from build123d import *

# Parameters (mm, degrees)
SKETCH1_W               = 100
SKETCH1_H               = 55
BOSS_EXTRUDE1_DEPTH     = 4
F_6_CLEARANCE_HOLE1_D   = 4.3053
SKETCH4_R               = 26
CUT_EXTRUDE1_DEPTH      = 1.5
BOSS_EXTRUDE2_DEPTH     = 2
CUT_EXTRUDE2_REACH      = 59.204
SKETCH7_W               = 22.5
SKETCH7_H               = 7
MIRROR2_COPY_1_DEPTH    = 2
MIRROR2_COPY_2_REACH    = 59.204
MIRROR2_COPY_2_SKETCH_W = 22.5
MIRROR2_COPY_2_SKETCH_H = 7
FILLET1_R               = 5


with BuildPart() as part:
    # Sketch1 → Boss-Extrude1 (new body)
    with BuildSketch(Plane(origin=(0, 0, 0), x_dir=(1, 0, 0), z_dir=(0, 1, 0))):
        Rectangle(SKETCH1_W, SKETCH1_H)
    extrude(amount=BOSS_EXTRUDE1_DEPTH)

    # #6 Clearance Hole1 (through all)
    with Locations(Plane(origin=(0, 4, 0), x_dir=(1, 0, 0), z_dir=(0, 1, 0))):
        with Locations((45.6352, 13.470384182), (45.6352, -13.470384182), (-46.825, -13.470384182), (-46.825, 13.470384182), (-20, 0)):
            Hole(F_6_CLEARANCE_HOLE1_D / 2)

    # Sketch4 → Cut-Extrude1 (cut)
    with BuildSketch(Plane(origin=(0, 4, 0), x_dir=(1, 0, 0), z_dir=(0, 1, 0))):
        with Locations(Location((0, 0, 0), (0, 0, 270))):
            Circle(SKETCH4_R)
    extrude(amount=-CUT_EXTRUDE1_DEPTH, mode=Mode.SUBTRACT)

    # Sketch6 → Boss-Extrude2 (add)
    with BuildSketch(Plane(origin=(0, 4, 0), x_dir=(1, 0, 0), z_dir=(0, 1, 0))):
        Polygon((-20.5, 25.5), (-20.5, 27.5), (-27.5, 27.5), (-27.5, 20.5), (-25.5, 20.5), (-25.5, 25.5), align=None)
    boss_extrude2 = extrude(amount=BOSS_EXTRUDE2_DEPTH)

    # Sketch7 → Cut-Extrude2 (cut, up to next)
    with BuildSketch(Plane(origin=(0, 4, 0), x_dir=(1, 0, 0), z_dir=(0, 1, 0)), mode=Mode.PRIVATE) as cut_extrude2_sk1:
        with Locations((-38.75, 24)):
            Rectangle(SKETCH7_W, SKETCH7_H)
    cut_extrude2_tool1 = extrude(cut_extrude2_sk1.sketch, amount=-CUT_EXTRUDE2_REACH, mode=Mode.PRIVATE) & part.part
    cut_extrude2 = cut_extrude2_tool1.solids().sort_by_distance((-38.75, 4, -24))[0]
    add(cut_extrude2, mode=Mode.SUBTRACT)

    # Mirror1: Boss-Extrude2, Cut-Extrude2 across plane
    add(boss_extrude2.mirror(Plane.XY))
    add(cut_extrude2.mirror(Plane.XY), mode=Mode.SUBTRACT)

    # Mirror2: Boss-Extrude2, Cut-Extrude2 across plane
    add(boss_extrude2.mirror(Plane(origin=(0, 0, 0), x_dir=(0, 0, 1), z_dir=(1, 0, 0))))
    add(cut_extrude2.mirror(Plane(origin=(0, 0, 0), x_dir=(0, 0, 1), z_dir=(1, 0, 0))), mode=Mode.SUBTRACT)

    # Mirror2 copy 1 sketch → Mirror2 copy 1 (add)
    with BuildSketch(Plane(origin=(0, 4, 0), x_dir=(-1, 0, 0), z_dir=(0, 1, 0))):
        Polygon((-20.5, 25.5), (-20.5, 27.5), (-27.5, 27.5), (-27.5, 20.5), (-25.5, 20.5), (-25.5, 25.5), align=None)
    extrude(amount=MIRROR2_COPY_1_DEPTH)

    # Mirror2 copy 2 sketch → Mirror2 copy 2 (cut, up to next)
    with BuildSketch(Plane(origin=(0, 4, 0), x_dir=(-1, 0, 0), z_dir=(0, 1, 0)), mode=Mode.PRIVATE) as mirror2_copy_2_sk1:
        with Locations((-38.75, 24)):
            Rectangle(MIRROR2_COPY_2_SKETCH_W, MIRROR2_COPY_2_SKETCH_H)
    mirror2_copy_2_tool1 = extrude(mirror2_copy_2_sk1.sketch, amount=-MIRROR2_COPY_2_REACH, mode=Mode.PRIVATE) & part.part
    add(mirror2_copy_2_tool1.solids().sort_by_distance((38.75, 4, 24))[0], mode=Mode.SUBTRACT)

    # Fillet1
    fillet1_edges = [part.edges().sort_by_distance(p)[0] for p in [
        (-50, 2, 20.5),
        (-27.5, 2, 20.5),
        (50, 2, 20.5),
        (27.5, 2, 20.5),
        (50, 2, -20.5),
        (27.5, 2, -20.5),
        (-50, 2, -20.5),
        (-27.5, 2, -20.5),
    ]]
    fillet(fillet1_edges, radius=FILLET1_R)


solid = part.part
Verification items for the finished model (mm, model axes). A direction names the side the tool comes from. Coordinates: 2 decimals unless noted, no trailing zeros. Write each loop counter-clockwise with the first axis right and the second up, starting at its lowest first coordinate (ties: lowest second). Pieces come first, ordered by that corner, then holes. Notation, with made-up numbers: M 28.5,-38.75 L 32.5,-38.75 A10 ccw 32.5,-25.75 Z; hole C -39,66 d9. An arc over 180 degrees is marked long. Use CSV: the item, a comma, the result in double quotes.
Q1. Section check B-B, the plane x = 0. Enter the section's corners in (y, z), and give its area (3 significant figures).
Computed values:
outline,"M 0,-27.5 L 4,-27.5 L 4,-26 L 2.5,-26 L 2.5,26 L 4,26 L 4,27.5 L 0,27.5 Z"
area,"142 mm²"
Q2. Section check A-A, the plane z = 0. Enter the section's corners in (x, y).
Computed values:
outline,"M -50,0 L -22.15,0 L -22.15,2.5 L -26,2.5 L -26,4 L -50,4 Z; M -17.85,0 L 50,0 L 50,4 L 26,4 L 26,2.5 L -17.85,2.5 Z"
Q3. Mould release check, pull along Z, two halves, no side actions. Record for faces 5 (the flat face through (-23, 4, -13)), 6 (the flat face through (26, 6, -25)), 7 (the cylindrical face through (-48.57, 1.97, -19)): pulls with the +Z half, pulls with the -Z half, needs draft (parallel to the pull), parting line crosses it, or undercut.
Computed values:
face 5,"undercut"
face 6,"needs draft"
face 7,"pulls with the -Z half"
Q4. Section check D-D, the plane z = -21.5. Enter the section's corners in (x, y), and give its area (3 significant figures).
Computed values:
outline,"M -29.5,0 L 29.5,0 L 29.5,4 L 27.5,4 L 27.5,6 L 25.5,6 L 25.5,4 L 14.62,4 L 14.62,2.5 L -14.62,2.5 L -14.62,4 L -25.5,4 L -25.5,6 L -27.5,6 L -27.5,4 L -29.5,4 Z"
area,"200 mm²"
Q5. Section check C-C, the plane z = 14.5. Enter the section's corners in (x, y), and give its area (3 significant figures).
Computed values:
outline,"M -50,0 L -48.72,0 L -48.72,4 L -50,4 Z; M -44.93,0 L 43.74,0 L 43.74,4 L 21.58,4 L 21.58,2.5 L -21.58,2.5 L -21.58,4 L -44.93,4 Z; M 47.53,0 L 50,0 L 50,4 L 47.53,4 Z"
area,"305 mm²"
Q6. Go/stop test with flat-tipped pins: P1, Ø2, axis at x = -35.5, y = 1, coming from the +Z side; P2, Ø1.6, axis at y = 4.5, z = 27, coming from the +X side; P3, Ø4, axis at x = 19.5, z = 16, coming from the +Y side. Record where each tip stops, or that it passes through.
Computed values:
P1,"z = 20.5"
P2,"x = 27.5"
P3,"y = 4"
Q7. Set-up check for faces 1 (the flat face through (-27, 5, 20.5)), 2 (the flat face through (-23, 5, -25.5)), 3 (the flat face through (-27.5, 4.4, 24.7)), 4 (the flat face through (-20.5, 5, -26)): record each of +Z, -Z, +X, -X, +Y, -Y from which the full face is reachable in a straight line by a thin tool's end or side.
Computed values:
face 1,"+X, -X, +Y"
face 2,"+Y"
face 3,"+Z, -X, +Y"
face 4,"+Z, -Z, +Y"
Q8. Thickness scan on line 1 along Z through (x, y) = (-20, 0.9); line 2 along X through (y, z) = (3.75, 0); line 3 along X through (y, z) = (3.1, 12.5). Record the ranges inside material, lowest first. Write a range as [from, to].
Computed values:
line 1,"[-27.5, -2.15], [2.15, 27.5]"
line 2,"[-50, -26], [26, 50]"
line 3,"[-50, -48.75], [-44.9, -22.8], [22.8, 43.71], [47.56, 50]"
